Part model, mm, in its own coordinate system. Give positions to 0.01 mm unless a question says otherwise; leave off trailing zeros. Order: outer loops, then holes, each group sorted by start corner. A loop starts at its lowest first (then second) coordinate and runs counter-clockwise, first axis right, second up. Notation, with made-up numbers: (89, -1.5) -> (126, -1.5) arc R10 ccw to (126, 2.5) -> close; hole circle Ø9 at (3, 27). An arc over 180 degrees is marked (long way). Write item = value, one per line. Start each with the question number.
Item 1: Band-saw the part on B-B on x = -42. Write the cut outline in (y, z).
Item 2: Band-saw the part on A-A on y = 41. Write the cut outline in (x, z), plus the area to 3 significant figures.
Item 3: Band-saw the part on C-C on z = 2.5. Count the separate pieces of the cut face and the enclosed holes in it, plus the area to 3 significant figures.
Item 4: Flat gauge pins, fed straight in: P1, Ø1.5, axis at y = -26.5, z = 2.5, coming from the -X side; P2, Ø0.9, axis at y = 32, z = 2, coming from the +X side; P3, Ø1.8, axis at x = 53.56, y = 48, coming from the +Z side. Where does each tip first touch, or does it go through?
Item 5: Drill centre lines: line 1 along Y through (x, z) = (-71, 1.3); line 2 along Y through (x, z) = (-68, 1.5); line 3 along Y through (x, z) = (10, 1.3). Where is each one in solid material? Low to high.
```python
from build123d import *

# Parameters (mm, degrees)
SKETCH3_W                                  = 114
SKETCH3_H                                  = 104
BOSS_EXTRUDE1_DEPTH                        = 3
SKETCH4_R                                  = 1.5
CUT_EXTRUDE1_DEPTH                         = 78.21398837
LPATTERN1_COUNT                            = 2
LPATTERN1_PITCH                            = 106.56
LPATTERN1_COUNT_DIR2                       = 2
LPATTERN1_PITCH_DIR2                       = 96.56
BOSS_EXTRUDE2_DEPTH                        = 3
SKETCH6_R                                  = 1.5
CUT_EXTRUDE2_DEPTH                         = 94.79232378
MIRROR1_AT_THE_SECOND_PLANE_COPY_1_DEPTH   = 3
MIRROR1_AT_THE_SECOND_PLANE_COPY_2_SKETC_R = 1.5
MIRROR1_AT_THE_SECOND_PLANE_COPY_2_DEPTH   = 94.79232378
CUT_EXTRUDE3_DEPTH                         = 94.79232378


with BuildPart() as part:
    # Sketch3 → Boss-Extrude1 (new body)
    with BuildSketch(Plane.XY):
        Rectangle(SKETCH3_W, SKETCH3_H)
    extrude(amount=BOSS_EXTRUDE1_DEPTH)

    # Sketch4 → Cut-Extrude1 (cut, through all)
    with BuildSketch(Plane.XY.offset(3)):
        with Locations((-53, 48)):
            Circle(SKETCH4_R)
    cut_extrude1 = extrude(amount=-CUT_EXTRUDE1_DEPTH, mode=Mode.SUBTRACT)

    # LPattern1: Cut-Extrude1 2 × 2
    with Locations(*[(i * LPATTERN1_PITCH, -j * LPATTERN1_PITCH_DIR2, 0) for i in range(LPATTERN1_COUNT) for j in range(LPATTERN1_COUNT_DIR2) if (i, j) != (0, 0)]):
        add(cut_extrude1, mode=Mode.SUBTRACT)

    # Sketch5 → Boss-Extrude2 (add)
    with BuildSketch(Plane.XY.offset(3)):
        with BuildLine():
            Line((-57, 52), (-71, 52))
            ThreePointArc((-71, 52), (-78, 45), (-71, 38))
            Line((-71, 38), (-57, 38))
            Line((-57, 38), (-57, 52))
        make_face()
    boss_extrude2 = extrude(amount=-BOSS_EXTRUDE2_DEPTH)

    # Sketch6 → Cut-Extrude2 (cut, through all)
    with BuildSketch(Plane.XY.offset(3)):
        with Locations((-71, 45)):
            Circle(SKETCH6_R)
    cut_extrude2 = extrude(amount=-CUT_EXTRUDE2_DEPTH, mode=Mode.SUBTRACT)

    # Mirror1: Boss-Extrude2, Cut-Extrude2 across plane
    add(boss_extrude2.mirror(Plane.ZX))
    add(cut_extrude2.mirror(Plane.ZX), mode=Mode.SUBTRACT)

    # Mirror1 at the second plane: Boss-Extrude2, Cut-Extrude2 across plane
    add(boss_extrude2.mirror(Plane(origin=(0, 0, 0), x_dir=(0, 0, 1), z_dir=(1, 0, 0))))
    add(cut_extrude2.mirror(Plane(origin=(0, 0, 0), x_dir=(0, 0, 1), z_dir=(1, 0, 0))), mode=Mode.SUBTRACT)

    # Mirror1 at the second plane copy 1 sketc → Mirror1 at the second plane copy 1 (add)
    with BuildSketch(Plane(origin=(0, 0, 3), x_dir=(-1, 0, 0), z_dir=(0, 0, 1))):
        with BuildLine():
            Line((-57, 52), (-71, 52))
            ThreePointArc((-71, 52), (-78, 45), (-71, 38))
            Line((-71, 38), (-57, 38))
            Line((-57, 38), (-57, 52))
        make_face()
    extrude(amount=-MIRROR1_AT_THE_SECOND_PLANE_COPY_1_DEPTH)

    # Mirror1 at the second plane copy 2 sketc → Mirror1 at the second plane copy 2 (cut, through all)
    with BuildSketch(Plane(origin=(0, 0, 3), x_dir=(-1, 0, 0), z_dir=(0, 0, 1))):
        with Locations((-71, 45)):
            Circle(MIRROR1_AT_THE_SECOND_PLANE_COPY_2_SKETC_R)
    extrude(amount=-MIRROR1_AT_THE_SECOND_PLANE_COPY_2_DEPTH, mode=Mode.SUBTRACT)

    # Sketch7 → Cut-Extrude3 (cut, through all)
    with BuildSketch(Plane.XY.offset(3)):
        Polygon((-2.72, -48), (-2.72, -6.740598429), (-48.517935743, -48), align=None)
        Polygon((49.077935743, -48), (3.28, -6.740598429), (3.28, -48), align=None)
        Polygon((53.56, -3), (8.092064257, -3), (53.56, -43.962104273), align=None)
        Polygon((53.56, 43.962104273), (8.092064257, 3), (53.56, 3), align=None)
        Polygon((3.28, 48), (3.28, 6.740598429), (49.077935743, 48), align=None)
        Polygon((-48.517935743, 48), (-2.72, 6.740598429), (-2.72, 48), align=None)
        Polygon((-53, 43.962104273), (-53, 3), (-7.532064257, 3), align=None)
        Polygon((-7.532064257, -3), (-53, -3), (-53, -43.962104273), align=None)
    extrude(amount=-CUT_EXTRUDE3_DEPTH, mode=Mode.SUBTRACT)


solid = part.part
```
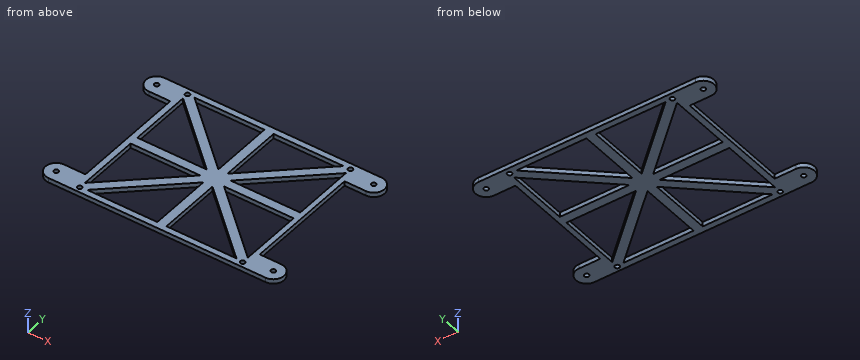
Values found:
q1.outline = (-52, 0) -> (-48, 0) -> (-48, 3) -> (-52, 3) -> close; (-42.13, 0) -> (-34.05, 0) -> (-34.05, 3) -> (-42.13, 3) -> close; (-3, 0) -> (3, 0) -> (3, 3) -> (-3, 3) -> close; (34.05, 0) -> (42.13, 0) -> (42.13, 3) -> (34.05, 3) -> close; (48, 0) -> (52, 0) -> (52, 3) -> (48, 3) -> close
q2.outline = (-76.74, 0) -> (-53, 0) -> (-53, 3) -> (-76.74, 3) -> close; (-49.71, 0) -> (-40.75, 0) -> (-40.75, 3) -> (-49.71, 3) -> close; (-2.72, 0) -> (3.28, 0) -> (3.28, 3) -> (-2.72, 3) -> close; (41.31, 0) -> (50.27, 0) -> (50.27, 3) -> (41.31, 3) -> close; (53.56, 0) -> (76.74, 0) -> (76.74, 3) -> (53.56, 3) -> close
q2.area = 213 mm^2
q3.separate_pieces = 1
q3.enclosed_holes = 16
q3.area = 5,390 mm^2
q4.P1 = -57
q4.P2 = 57
q4.P3 = through
q5.line_1 = -52 to -46.5, -43.5 to -38, 38 to 43.5, 46.5 to 52
q5.line_2 = -52 to -38, 38 to 52
q5.line_3 = -52 to -48, -12.79 to -4.72, -3 to 3, 4.72 to 12.79, 48 to 52
